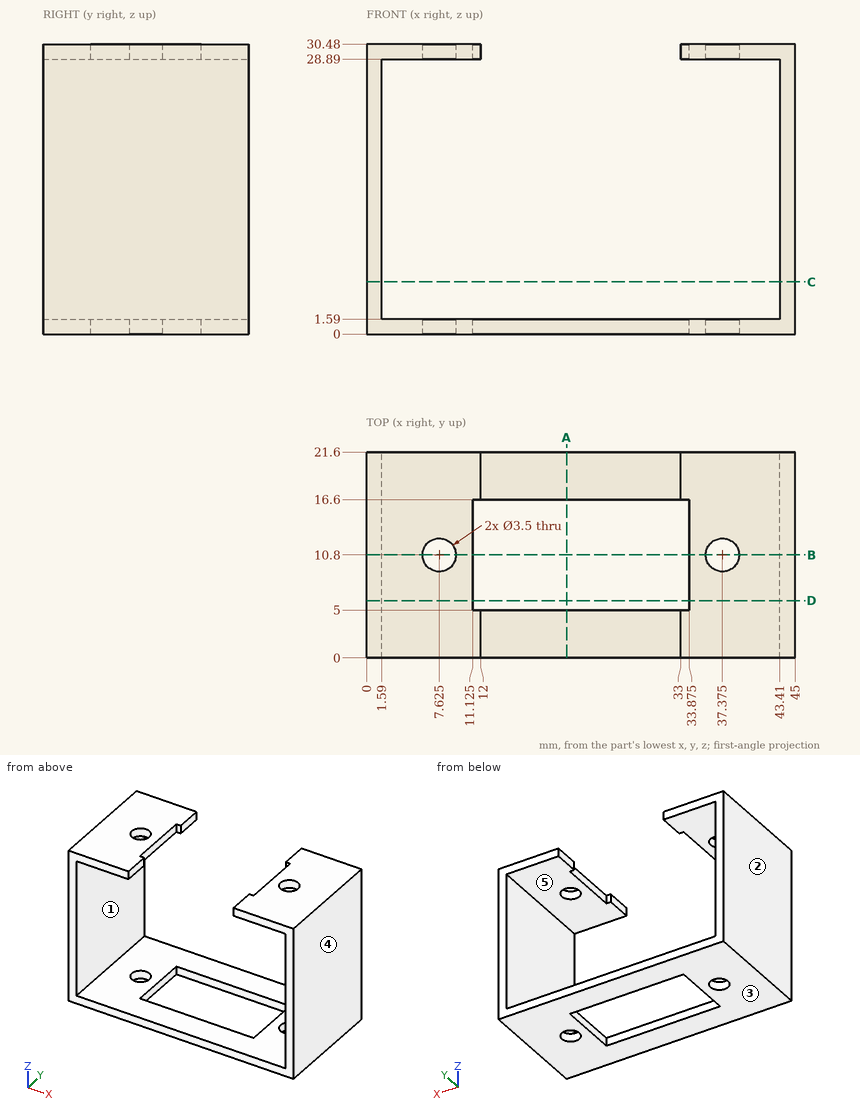
Could you check a few things on this drawing? It's one solid part, dimensions in mm from its lowest x, y, z. A direction names the side the tool comes from. Give positions to 0.01 mm unless a question says otherwise; leave off trailing zeros. Order: outer loops, then holes, each group sorted by start corner. A loop starts at its lowest first (then second) coordinate and runs counter-clockwise, first axis right, second up. Notation, with made-up numbers: (66, 40.5) - (88, 40.5) arc R19 cw to (88, 58.5) - close; hole circle Ø5 at (15, -0.5). An arc over 180 degrees is marked (long way). Return JSON: item names as keys, results as strings. Group by question number.
Q1. Suppose I cut it at C-C, the plane z = 5.5. Please give me the cut outline in (x, y).
Q2. Suppose I cut it at B-B, the plane y = 10.8. State how many separate pieces and enclosed holes the cut face has, and give its area (3 significant figures).
Q3. Please list where these lines run through material, in increasing order: line 1 along Y through (x, z) = (37.5, 29); line 2 along Z through (x, y) = (36, 6.25); line 3 along X through (y, z) = (17.25, 23.5). Write a range as [from, to].
Q4. Will this pin go through, and if not, where does the flat tip stop? pin 1 Ø6.5 at (x, y) = (24, 7.5) entering from +Z.
Q5. Which directions (+Z, -Z, +X, -X, +Y, -Y) give clear straight access to the entire face, cutting with the end or side of a thin tool? Please do the marked faces 4 and 5.
Q6. Suppose I cut it at A-A, the plane x = 21. Please give me the cut outline in (y, z).
Q7. Suppose I cut it at D-D, the plane y = 6. Please give me the cut outline in (x, z) (3 decimals), and give its area (3 significant figures).
Q8. Thinking about a two-plate mould opening in Z: for the marked faces 1, 2 and 3, which applies, pulls with the +Z half, pulls with the -Z half, needs draft (parallel to the pull), parting line crosses it, or undercut?
Resolved:
{
 "1": {"outline": "(0, 0) - (1.59, 0) - (1.59, 21.6) - (0, 21.6) - close; (43.41, 0) - (45, 0) - (45, 21.6) - (43.41, 21.6) - close"},
 "2": {"separate pieces": "6", "enclosed holes": "0", "area": "135 mm2"},
 "3": {"line 1": "y = [0, 9.05], [12.55, 21.6]", "line 2": "z = [0, 1.59], [28.89, 30.48]", "line 3": "x = [0, 1.59], [43.41, 45]"},
 "4": {"pin 1": "stops at z = 1.59"},
 "5": {"face 4": "+Z, -Z, +X, +Y, -Y", "face 5": "+Y, -Y"},
 "6": {"outline": "(0, 0) - (5, 0) - (5, 1.59) - (0, 1.59) - close; (16.6, 0) - (21.6, 0) - (21.6, 1.59) - (16.6, 1.59) - close"},
 "7": {"outline": "(0, 0) - (11.125, 0) - (11.125, 1.59) - (1.59, 1.59) - (1.59, 28.89) - (11.125, 28.89) - (11.125, 30.48) - (0, 30.48) - close; (33.875, 0) - (45, 0) - (45, 30.48) - (33.875, 30.48) - (33.875, 28.89) - (43.41, 28.89) - (43.41, 1.59) - (33.875, 1.59) - close", "area": "158 mm2"},
 "8": {"face 1": "undercut", "face 2": "needs draft", "face 3": "pulls with the -Z half"}
}
